```python
from build123d import *

# Parameters (mm, degrees)
SKETCH2_W                                       = 35
SKETCH2_H                                       = 34
SKETCH2_W_2                                     = 30
SKETCH2_R                                       = 2
BOSS_EXTRUDE1_DEPTH                             = 10
FILLET1_R                                       = 1
CSK_FOR_M4_FLAT_HEAD_MACHINE_SCREW1_D           = 4.5
CSK_FOR_M4_FLAT_HEAD_MACHINE_SCREW1_DEPTH       = 10
CSK_FOR_M4_FLAT_HEAD_MACHINE_SCREW1_CSINK_D     = 9.4
CSK_FOR_M4_FLAT_HEAD_MACHINE_SCREW1_CSINK_ANGLE = 90
SKETCH3_R                                       = 4
BOSS_EXTRUDE2_DEPTH                             = 14
F_3_0MM_DOWEL_HOLE1_D                           = 3
F_3_0MM_DOWEL_HOLE1_DEPTH                       = 18.33030278
CUT_EXTRUDE1_DEPTH                              = 25
CSK_FOR_M3_FLAT_HEAD_MACHINE_SCREW1_D           = 3.4
CSK_FOR_M3_FLAT_HEAD_MACHINE_SCREW1_DEPTH       = 10
CSK_FOR_M3_FLAT_HEAD_MACHINE_SCREW1_CSINK_D     = 6.3
CSK_FOR_M3_FLAT_HEAD_MACHINE_SCREW1_CSINK_ANGLE = 90
CSK_FOR_M3_FLAT_HEAD_MACHINE_SCREW1_TIP         = 1.021463052
SKETCH15_W                                      = 29
SKETCH15_H                                      = 34
BOSS_EXTRUDE3_DEPTH                             = 35
SKETCH16_R                                      = 14.325
BOSS_EXTRUDE4_DEPTH                             = 15
BOSS_EXTRUDE5_DEPTH                             = 34


with BuildPart() as part:
    # Sketch2 → Boss-Extrude1 (new body)
    with BuildSketch(Plane(origin=(0, 0, 0), x_dir=(1, 0, 0), z_dir=(0, 1, 0))):
        with Locations((23.5, -12)):
            Rectangle(SKETCH2_W, SKETCH2_H)
        with Locations((-9, -12)):
            Rectangle(SKETCH2_W_2, SKETCH2_H)
        with Locations((0, -24)):
            Circle(SKETCH2_R, mode=Mode.SUBTRACT)
        with Locations((-18, -24)):
            Circle(SKETCH2_R, mode=Mode.SUBTRACT)
        with Locations((-18, 0)):
            Circle(SKETCH2_R, mode=Mode.SUBTRACT)
        Circle(SKETCH2_R, mode=Mode.SUBTRACT)
    boss_extrude1 = extrude(amount=BOSS_EXTRUDE1_DEPTH)

    # Fillet1
    fillet1_edges = [part.edges().sort_by_distance(p)[0] for p in [
        (-24, 5, 29),
        (-24, 5, -5),
    ]]
    fillet(fillet1_edges, radius=FILLET1_R)

    # CSK for M4 Flat Head Machine Screw1
    with Locations(Plane(origin=(0, 10, 0), x_dir=(1, 0, 0), z_dir=(0, 1, 0))):
        with Locations((-18, 0), (0, 0), (0, -24), (-18, -24)):
            csk_for_m4_flat_head_machine_screw1 = CounterSinkHole(CSK_FOR_M4_FLAT_HEAD_MACHINE_SCREW1_D / 2, CSK_FOR_M4_FLAT_HEAD_MACHINE_SCREW1_CSINK_D / 2, depth=CSK_FOR_M4_FLAT_HEAD_MACHINE_SCREW1_DEPTH, counter_sink_angle=CSK_FOR_M4_FLAT_HEAD_MACHINE_SCREW1_CSINK_ANGLE)

    # Sketch3 → Boss-Extrude2 (add)
    with BuildSketch(Plane.XY.offset(19)):
        with BuildLine():
            ThreePointArc((-18.974091996, 16.203347698), (-19.957675635, 12.488863747), (-22.885197632, 10))
            Line((-22.885197632, 10), (4.885197632, 10))
            ThreePointArc((4.885197632, 10), (1.957675635, 12.488863747), (0.974091996, 16.203347698))
            ThreePointArc((0.974091996, 16.203347698), (0.979733938, 16.309510649), (0.987131717, 16.415565714))
            ThreePointArc((0.987131717, 16.415565714), (0.837737799, 18.716848177), (0.16515139, 20.922714683))
            Line((0.16515139, 20.922714683), (0.16515139, 27.923199435))
            Line((0.16515139, 27.923199435), (-18.16515139, 27.923199435))
            Line((-18.16515139, 27.923199435), (-18.16515139, 20.922714683))
            ThreePointArc((-18.16515139, 20.922714683), (-18.837737799, 18.716848177), (-18.987131717, 16.415565714))
            ThreePointArc((-18.987131717, 16.415565714), (-18.979733938, 16.309510649), (-18.974091996, 16.203347698))
        make_face()
        with Locations((-9, 16.922714683)):
            Circle(SKETCH3_R, mode=Mode.SUBTRACT)
    boss_extrude2 = extrude(amount=-BOSS_EXTRUDE2_DEPTH)

    # Ø3.0mm Dowel Hole1
    with Locations(Plane(origin=(0.16515139, 0, 0), x_dir=(0, 0, -1), z_dir=(1, 0, 0))):
        with Locations((-16, 23.923199435), (-8, 23.923199435)):
            f_3_0mm_dowel_hole1 = Hole(F_3_0MM_DOWEL_HOLE1_D / 2, depth=F_3_0MM_DOWEL_HOLE1_DEPTH)

    # Sketch10 → Cut-Extrude1 (cut, through all)
    with BuildSketch(Plane.XY.offset(19)):
        with BuildLine():
            Line((-9, 27.923199435), (-10, 27.923199435))
            Line((-10, 27.923199435), (-10, 20.795698029))
            ThreePointArc((-10, 20.795698029), (-9.50401717, 20.890833468), (-9, 20.922714683))
            Line((-9, 20.922714683), (-9, 27.923199435))
        make_face()
        with BuildLine():
            Line((-8, 27.923199435), (-9, 27.923199435))
            Line((-9, 27.923199435), (-9, 20.922714683))
            ThreePointArc((-9, 20.922714683), (-8.49598283, 20.890833468), (-8, 20.795698029))
            Line((-8, 20.795698029), (-8, 27.923199435))
        make_face()
    cut_extrude1 = extrude(amount=-CUT_EXTRUDE1_DEPTH, mode=Mode.SUBTRACT)

    # Mirror11: Boss-Extrude1, CSK for M4 Flat Head Machine Screw1, Boss-Extrude2, Ø3.0mm Dowel Hole1, Cut-Extrude1 across plane
    add(boss_extrude1.mirror(Plane(origin=(41, 10, 0), x_dir=(0, 0, 1), z_dir=(1, 0, 0))))
    add(csk_for_m4_flat_head_machine_screw1.mirror(Plane(origin=(41, 10, 0), x_dir=(0, 0, 1), z_dir=(1, 0, 0))), mode=Mode.SUBTRACT)
    add(boss_extrude2.mirror(Plane(origin=(41, 10, 0), x_dir=(0, 0, 1), z_dir=(1, 0, 0))))
    add(f_3_0mm_dowel_hole1.mirror(Plane(origin=(41, 10, 0), x_dir=(0, 0, 1), z_dir=(1, 0, 0))), mode=Mode.SUBTRACT)
    add(cut_extrude1.mirror(Plane(origin=(41, 10, 0), x_dir=(0, 0, 1), z_dir=(1, 0, 0))), mode=Mode.SUBTRACT)

    # CSK for M3 Flat Head Machine Screw1
    with Locations(Plane(origin=(0, 0, -5), x_dir=(-1, 0, 0), z_dir=(0, 0, -1))):
        with Locations((-69.114802368, 5), (-59.114802368, 5), (-13.885197632, 5), (-23.885197632, 5)):
            CounterSinkHole(CSK_FOR_M3_FLAT_HEAD_MACHINE_SCREW1_D / 2, CSK_FOR_M3_FLAT_HEAD_MACHINE_SCREW1_CSINK_D / 2, depth=CSK_FOR_M3_FLAT_HEAD_MACHINE_SCREW1_DEPTH, counter_sink_angle=CSK_FOR_M3_FLAT_HEAD_MACHINE_SCREW1_CSINK_ANGLE)
            with Locations((0, 0, -(CSK_FOR_M3_FLAT_HEAD_MACHINE_SCREW1_DEPTH + CSK_FOR_M3_FLAT_HEAD_MACHINE_SCREW1_TIP / 2))):  # 118° drill point
                Cone(0, CSK_FOR_M3_FLAT_HEAD_MACHINE_SCREW1_D / 2, CSK_FOR_M3_FLAT_HEAD_MACHINE_SCREW1_TIP, mode=Mode.SUBTRACT)

    # Sketch15 → Boss-Extrude3 (add)
    with BuildSketch(Plane(origin=(0, 0, 0), x_dir=(1, 0, 0), z_dir=(0, 1, 0))):
        with Locations((120.5, -12)):
            Rectangle(SKETCH15_W, SKETCH15_H)
    extrude(amount=BOSS_EXTRUDE3_DEPTH)

    # Sketch16 → Boss-Extrude4 (add)
    with BuildSketch(Plane(origin=(0, 35, 0), x_dir=(1, 0, 0), z_dir=(0, 1, 0))):
        Polygon((103.982508934, -29), (135, -29), (135, 5), (103.982508934, 5), (103.982508934, -11.839034668), align=None)
        with Locations((118.6, -11.839034668)):
            Circle(SKETCH16_R, mode=Mode.SUBTRACT)
    extrude(amount=BOSS_EXTRUDE4_DEPTH)

    # Sketch17 → Boss-Extrude5 (add)
    with BuildSketch(Plane.XY.offset(29)):
        Polygon((103.982508934, 35), (106, 30), (106, 35), align=None)
    extrude(amount=-BOSS_EXTRUDE5_DEPTH)


solid = part.part
```
Check sheet for the modelled part. Datum: model origin and axes. Units: mm. A direction names the side the tool comes from. Coordinates: 2 decimals unless noted, no trailing zeros. Order: outer loops, then holes, each group sorted by start corner. A loop starts at its lowest first (then second) coordinate and runs counter-clockwise, first axis right, second up. Notation, with made-up numbers: (47.5, 10.25) -> (59.5, 10.25) arc R10 cw to (59.5, 23.25) -> close; hole circle Ø6 at (81, -11). An arc over 180 degrees is marked (long way). Write each question's results on one line, items separated by ' | '. Start each with the question number.
1) Draft check along Z on faces 1 (the face through (107.232, 42.395, 20.556)), 2 (the face through (12.536, 3.966, 0.785)), 3 (the face through (96.14, 23.01, 14.81)). Enter one of: pulls with the +Z half, pulls with the -Z half, needs draft (parallel to the pull), parting line crosses it, or undercut.
2) Section check C-C (x = 54). Enter the section's corners in (y, z), and give its area (3 significant figures).
3) Material ranges on line 1 along X through (y, z) = (6.5, 24); line 2 along Z through (x, y) = (82, 5.5); line 3 along Z through (x, y) = (-13, 23.5), recorded low to high.
4) Depth check by flat-ended pin: pin 1 (7 mm diameter, centred on x = -9, y = 16.92, fed in from -Z); pin 2 (10 mm diameter, centred on x = 88, y = 14, fed in from +Z); pin 3 (6 mm diameter, centred on y = 20.5, z = 4.5, fed in from -X); pin 4 (3 mm diameter, centred on x = 39.5, z = 22, fed in from +Y). Enter the tip coordinate at first touch or a pass-through.
5) Set-up check for faces 4 (the face through (86, 27.923, 12)), 5 (the face through (100.165, 24, 12)), 6 (the face through (106, 20, 12)), 7 (the face through (104.98, 32.53, 12.24)): record each of +Z, -Z, +X, -X, +Y, -Y from which the full face is reachable in a straight line by a thin tool's end or side.
6) Section check A-A (x = 93.5). Enter the section's corners in (y, z), and give its area (3 significant figures).
7) Section check B-B (z = 0). Count the separate pieces of the cut face and the enclosed holes in it, and give its area (3 significant figures).
Checked values:
1) face 1: undercut | face 2: needs draft | face 3: undercut
2) outline: (0, -5) -> (10, -5) -> (10, 29) -> (0, 29) -> close | area: 340 mm²
3) line 1: -24 to -20.25, -15.75 to -2.25, 2.25 to 79.75, 84.25 to 97.75, 102.25 to 135 | line 2: -5 to -2.25, 2.25 to 21.75, 26.25 to 29 | line 3: 5 to 6.56, 9.44 to 14.56, 17.44 to 19
4) pin 1: through | pin 2: z = 29 | pin 3: x = -18.98 | pin 4: y = 10
5) face 4: +Z, -Z, -X, +Y | face 5: +Z, -Z, +Y | face 6: +Z, -Z | face 7: +Z, -Z, -X
6) outline: (0, -5) -> (10, -5) -> (10, 5) -> (13.8, 5) -> (13.8, 19) -> (10, 19) -> (10, 29) -> (0, 29) -> close; (20.05, 5) -> (27.92, 5) -> (27.92, 19) -> (20.05, 19) -> close; hole circle Ø3 at (23.92, 8); hole circle Ø3 at (23.92, 16) | area: 489 mm²
7) separate pieces: 5 | enclosed holes: 4 | area: 2,300 mm²
